The listing builds one solid part. Answer for the finished solid, in the listing's coordinates (mm). A direction names the side the tool comes from. Coordinates: 2 decimals unless noted, no trailing zeros. Loops run counter-clockwise (first coordinate to the right, second up) from the corner with the lowest first, then second, coordinate; pieces in that order, holes last. Notation, with made-up numbers: M 33.5,83.5 L 68.5,83.5 A21 cw 68.5,89.5 Z; hole C 4.5,85 d10. An arc over 180 degrees is marked long. Return JSON: item names as keys, results as strings. Group by question number.
1. Section A-A (y = -0.5) is taken. Write down the section's boundary in (x, z).
2. Section D-D (y = 0.95) is taken. Write down the section's boundary in (x, z), then the cut area to 3 significant figures.
3. Section C-C (z = 2.25) is taken. Write down the section's boundary in (x, y).
4. Which of the six approach directions +Z, -Z, +X, -X, +Y, -Y give full straight-line access (tool end or side, diameter ignored) to faces 1 (the face through (4, 0, 0)), 2 (the face through (5.25, -0.5, -1.4)), 3 (the face through (2.75, 1, -1)), 4 (the face through (-2.75, 1, 1)), 5 (the face through (-1.92, 0.99, -1.97))?
5. Given P1, Ø0.6, axis at y = 0.5, z = -1.5, coming from the +X side; P2, Ø1.6, axis at y = 0.5, z = 1, coming from the -X side; P3, Ø1.5, axis at x = -4, z = 0, coming from the +Y side, each flat-ended and moving along its own axis, determine where each tip first touches the part or whether it passes through.
6. Straight lines are drawn through the part: L1, parallel to Z at x = 0, y = 1.1; L2, parallel to X at y = 1.25, z = -1.25. For each, find the intervals that lie inside material, in ascending order. Write a range as from..to.
```python
from build123d import *
from build123d import SkipClean  # not in build123d's __all__

# Parameters (mm, degrees)
F0_R     = 1.5
F1_DEPTH = 3.8
F3_DEPTH = 2
F5_DEPTH = 25
F6_W     = 5.9742073228
F6_H     = 0.5
F7_DEPTH = 25


# Not quite as in the source:
# - after a boolean that leaves OpenCascade's solid faulty, fix() repairs it


with BuildPart() as f1:
    # F0 (on Front) → F1 (new body)
    with BuildSketch(Plane.XZ):
        with BuildLine():
            Line((-4.472135955, -2.75), (4.472135955, -2.75))
            ThreePointArc((4.472135955, -2.75), (5.0517924425, -1.4289482559), (5.25, 0))
            ThreePointArc((5.25, 0), (5.0517924425, 1.4289482559), (4.472135955, 2.75))
            Line((4.472135955, 2.75), (-4.472135955, 2.75))
            ThreePointArc((-4.472135955, 2.75), (-5.0517924425, 1.4289482559), (-5.25, 0))
            ThreePointArc((-5.25, 0), (-5.0517924425, -1.4289482559), (-4.472135955, -2.75))
        make_face()
        Circle(F0_R, mode=Mode.SUBTRACT)
        with BuildLine():
            Line((-5.25, 2.75), (-5.25, 0))
            ThreePointArc((-5.25, 0), (-5.0517924425, 1.4289482559), (-4.472135955, 2.75))
            Line((-4.472135955, 2.75), (-5.25, 2.75))
        make_face()
        with BuildLine():
            Line((4.472135955, -2.75), (5.25, -2.75))
            Line((5.25, -2.75), (5.25, 0))
            ThreePointArc((5.25, 0), (5.0517924425, -1.4289482559), (4.472135955, -2.75))
        make_face()
    extrude(amount=F1_DEPTH)

    # F2 (on face) → F3 (join)
    with BuildSketch(Plane(origin=(0, 0, 0), x_dir=(-1, 0, 0), z_dir=(0, 1, 0))):
        with BuildLine():
            Line((1.5, 0), (2.75, 0))
            ThreePointArc((2.75, 0), (1.9445436483, 1.9445436483), (0, 2.75))
            ThreePointArc((0, 2.75), (-1.9445436483, 1.9445436483), (-2.75, 0))
            Line((-2.75, 0), (-1.5, 0))
            ThreePointArc((-1.5, 0), (0, 1.5), (1.5, 0))
        make_face()
        with BuildLine():
            ThreePointArc((0, -2.75), (1.9445436483, -1.9445436483), (2.75, 0))
            Line((2.75, 0), (1.5, 0))
            ThreePointArc((1.5, 0), (0, -1.5), (-1.5, 0))
            Line((-1.5, 0), (-2.75, 0))
            ThreePointArc((-2.75, 0), (-1.9445436483, -1.9445436483), (0, -2.75))
        make_face()
        with BuildLine():
            ThreePointArc((0, 2.75), (1.9445436483, 1.9445436483), (2.75, 0))
            Line((2.75, 0), (2.75, 2.75))
            Line((2.75, 2.75), (0, 2.75))
        make_face()
        with BuildLine():
            Line((-2.75, -2.75), (0, -2.75))
            ThreePointArc((0, -2.75), (-1.9445436483, -1.9445436483), (-2.75, 0))
            Line((-2.75, 0), (-2.75, -2.75))
        make_face()
    with SkipClean():  # cleaning this boolean's faces spoils the solid; the shape is the same uncleaned
        extrude(amount=F3_DEPTH)

    # F4 (on face) → F5 (cut)
    with BuildSketch(Plane.XY.offset(2.75)):
        Polygon((-5.25, -1.1), (-5.25, -3.8), (-2.25, -3.8), align=None)
        Polygon((2.25, -3.8), (5.25, -3.8), (5.25, -1.1), align=None)
    extrude(amount=-F5_DEPTH, mode=Mode.SUBTRACT)

    add(f1.part.fix(), mode=Mode.REPLACE)

    # F6 (on face) → F7 (cut)
    with BuildSketch(Plane.XY.offset(2.75)):
        with Locations((-0.0664879346, -3.55)):
            Rectangle(F6_W, F6_H)
    extrude(amount=-F7_DEPTH, mode=Mode.SUBTRACT)


solid = f1.part
```
Worked out:
{
 "1": {"outline": "M -5.25,0 A5.25 ccw -4.47,-2.75 L 5.25,-2.75 L 5.25,0 A5.25 ccw 4.47,2.75 L -5.25,2.75 Z; hole C 0,0 d3"},
 "2": {"outline": "M -2.75,0 A2.75 ccw 0,-2.75 L 2.75,-2.75 L 2.75,0 A2.75 ccw 0,2.75 L -2.75,2.75 Z; hole C 0,0 d3", "area": "19.9 mm^2"},
 "3": {"outline": "M -5.25,-1.1 L -2.81,-3.3 L 2.81,-3.3 L 4.74,-1.56 L 4.74,0 L 1.58,0 L 1.58,2 L -2.75,2 L -2.75,0 L -5.25,0 Z"},
 "4": {"face 1": "+Z, +X, +Y", "face 2": "+Z, -Z, +X, +Y, -Y", "face 3": "+Z, -Z, +X, +Y", "face 4": "+Z, -Z, -X, +Y", "face 5": "-Z, -X, +Y"},
 "5": {"P1": "x = 2.75", "P2": "x = -5.25", "P3": "y = 0"},
 "6": {"L1": "-2.75..-1.5, 1.5..2.75", "L2": "-2.45..-0.83, 0.83..2.75"}
}
